Design review of the part built by this model. Coordinates are the model's own, in mm. A direction names the side the tool comes from. Give positions to 0.01 mm unless a question says otherwise; leave off trailing zeros. Write each loop counter-clockwise with the first axis right and the second up, starting at its lowest first coordinate (ties: lowest second). Pieces come first, ordered by that corner, then holes. Notation, with made-up numbers: M 81,18 L 88,18 A33 cw 88,47 Z; hole C 75,79.5 d1. An arc over 180 degrees is marked long. One line per item, written item: value. Start each with the question number.
```python
from build123d import *

# Parameters (mm, degrees)
F1_DEPTH  = 17
F2_W      = 26
F2_H      = 16
F3_DEPTH  = 44
F4_W      = 18
F4_H      = 25
F5_DEPTH  = 12
F8_DEPTH  = 17.5
F9_R      = 8
F10_R     = 10
F11_DEPTH = 25


# Not quite as in the source:
# - the program builds the solid bodies; features that only make, move or delete a surface that nothing else refers to are left out


with BuildPart() as f1:
    # F0 (on Front) → F1 (new body)
    with BuildSketch(Plane.XZ):
        Polygon((52.0617456436, 19.5316821036), (37.0617456436, 29.5316821036), (-26.9382543564, 29.5316821036), (-41.9382543564, 19.5316821036), (-41.9382543564, 13.5316821036), (52.0617456436, 13.5316821036), align=None)
    extrude(amount=F1_DEPTH)

    # F2 (on face) → F3 (join)
    with BuildSketch(Plane.XZ.offset(17)):
        with Locations((5.0617456436, 21.5316821036)):
            Rectangle(F2_W, F2_H)
    extrude(amount=F3_DEPTH)

    # F4 (on face) → F5 (cut)
    with BuildSketch(Plane.XY.offset(29.5316821036)):
        with Locations((5.0617456436, -48.5)):
            Rectangle(F4_W, F4_H)
        with BuildLine():
            Line((-3.9382543564, -36), (14.0617456436, -36))
            ThreePointArc((14.0617456436, -36), (5.0617456436, -27), (-3.9382543564, -36))
        make_face()
    extrude(amount=-F5_DEPTH, mode=Mode.SUBTRACT)

    # F7 (on offset) → F8 (join, symmetric)
    with BuildSketch(Plane.YZ.offset(5.0617456436)):
        Polygon((-17, 45.5316821036), (-17, 29.5316821036), (0, 29.5316821036), (0, 35.5316821036), (35, 35.5316821036), (35, 55.5316821036), (25, 55.5316821036), (25, 45.5316821036), align=None)
    extrude(amount=F8_DEPTH, both=True)

    # F9
    f9_edges = [f1.edges().sort_by_distance(p)[0] for p in [
        (5.061746, -17, 45.531682),
    ]]
    fillet(f9_edges, radius=F9_R)

    # F10 (on face) → F11 (cut)
    with BuildSketch(Plane.XY.offset(45.5316821036)):
        with Locations((5.0617456436, 12.5)):
            Circle(F10_R)
    extrude(amount=-F11_DEPTH, mode=Mode.SUBTRACT)


solid = f1.part
```
Q1. Take a section at C-C, the plane y = -39. Give the boundary of the cut face in (x, z), then the cut area to 3 significant figures.
Q2. Wall thickness on line 1 (X direction, y = 12, z = 39); line 2 (Z direction, x = 16.5, y = -57); line 3 (Z direction, x = 18, y = 15.5): over which ranges is each line inside the solid? List them lowest first. Write a range as from..to.
Q3. Take a section at A-A, the plane y = 12.5. Give the boundary of the cut face in (x, z).
Q4. Take a section at D-D, the plane z = 21.5. Give the boundary of the cut face in (x, y).
Q5. For P1, Ø6, axis at y = -46, z = 21.5, coming from the +X side; P2, Ø9.5, axis at y = -51.5, z = 25.5, coming from the -X side; P3, Ø16, axis at x = -19.5, y = -10, coming from the +Z side, all flat-tipped, find the tip position at first contact; note any pin that passes through.
Q6. The part is to be moulded in two halves that separate along X. For faces 5 (the face through (6, -17, 31)), 6 (the face through (18.062, -39, 21)), 7 (the face through (5, -44, 17.532)), say which applies: pulls with the +X half, pulls with the -X half, needs draft (parallel to the pull), parting line crosses it, or undercut.
Q7. Take a section at B-B, the plane x = 1. Give the boundary of the cut face in (y, z).
Q8. Machinability: for faces 1 (the face through (-7.938, -39, 21)), 2 (the face through (11, -29, 29.532)), 3 (the face through (5, -27, 24)), 4 (the face through (6, 0, 22)), which of the approach directions +Z, -Z, +X, -X, +Y, -Y give a long, thin tool a straight path to every point of the face, cutting with its end or side? Answer none if there is none.
Results list:
1. outline: M -7.94,13.53 L 18.06,13.53 L 18.06,29.53 L 14.06,29.53 L 14.06,17.53 L -3.94,17.53 L -3.94,29.53 L -7.94,29.53 Z
1. area: 200 mm^2
2. line 1: x = -12.44..-4.93, 15.05..22.56
2. line 2: z = 13.53..29.53
2. line 3: z = 35.53..45.53
3. outline: M -12.44,35.53 L -4.94,35.53 L -4.94,45.53 L -12.44,45.53 Z; M 15.06,35.53 L 22.56,35.53 L 22.56,45.53 L 15.06,45.53 Z
4. outline: M -38.99,-17 L -7.94,-17 L -7.94,-61 L -3.94,-61 L -3.94,-36 A9 cw 14.06,-36 L 14.06,-61 L 18.06,-61 L 18.06,-17 L 49.11,-17 L 49.11,0 L -38.99,0 Z
5. P1: stops at x = 18.06
5. P2: stops at x = -7.94
5. P3: stops at z = 45.53
6. face 5: needs draft
6. face 6: pulls with the +X half
6. face 7: undercut
7. outline: M -61,13.53 L 0,13.53 L 0,35.53 L 3.36,35.53 L 3.36,45.53 L -9,45.53 A8 ccw -17,37.53 L -17,29.53 L -27.97,29.53 L -27.97,17.53 L -61,17.53 Z; M 21.64,35.53 L 35,35.53 L 35,55.53 L 25,55.53 L 25,45.53 L 21.64,45.53 Z
8. face 1: +Z, -Z, -X, -Y
8. face 2: +Z, +X, -X, -Y
8. face 3: +Z, -Y
8. face 4: -Z, +X, -X, +Y
